The listing builds one solid part. Answer for the finished solid, in the listing's coordinates (mm). A direction names the side the tool comes from. Give positions to 0.01 mm unless a question says otherwise; leave off trailing zeros. Order: outer loops, then holes, each group sorted by start corner. A loop starts at its lowest first (then second) coordinate and runs counter-clockwise, first axis right, second up. Notation, with made-up numbers: (19.5, -35.75) - (69.5, -35.75) arc R22 ccw to (69.5, -17.75) - close; hole circle Ø10 at (53, 66.25). An arc over 180 degrees is marked (long way). Use a Markdown table: item, result. Add a question column.
1) The mould has two halves that part along X. Classify faces 4 (the face through (15, 0, 2)), 5 (the face through (13.953, 18.192, 2.348)), 6 (the face through (6.35, 2, 2)): released by +X, released by -X, zero draft, split by the parting line, or undercut.
2) Find section A-A, the plane y = 32. Determine the outline of the cut face in (x, z), plus the area to 3 significant figures.
3) Find section D-D, the plane y = 17.5. Determine the outline of the cut face in (x, z), plus the area to 3 significant figures.
4) Flat-ended cylindrical pins translate along their axes: pin 1 (2.5 mm diameter, centred on y = 30.5, z = 2, fed in from +X); pin 2 (1.4 mm diameter, centred on x = 0.5, z = 3, fed in from +Y); pin 3 (1.4 mm diameter, centred on y = 3, z = 2.5, fed in from -X). Find the tip coordinate at first contact, or state that the pin passes through.
5) Find section B-B, the plane z = 3.35. Determine the outline of the cut face in (x, y), plus the area to 3 significant figures.
6) For faces 1 (the face through (-6.35, 2, 2)), 2 (the face through (0, 25.722, 2)), 3 (the face through (-15, 0, 2)), determine the directions among +Z, -Z, +X, -X, +Y, -Y from which every point of the face is accessible in a straight line to the end or side of a thin tool.
7) Straight lines are drawn through the part: line 1 (Y direction, x = -1.5, z = 1.5); line 2 (X direction, y = 30, z = 0.25); line 3 (X direction, y = 27, z = 2.05). For each, find the intervals that lie inside material, in ascending order.
8) Find section C-C, the plane x = 1. Determine the outline of the cut face in (y, z), plus the area to 3 significant figures.
from build123d import *

# Parameters (mm, degrees)
BOSS_EXTRUDE1_DEPTH = 4.7625
CUT_EXTRUDE1_DEPTH  = 50.252795761
SKETCH4_W           = 4.7625
SKETCH4_H           = 4.7625
CUT_EXTRUDE2_DEPTH  = 10.16


with BuildPart() as part:
    # Sketch1 → Boss-Extrude1 (new body)
    with BuildSketch(Plane.XY):
        Polygon((0, 42.527367988), (24.384, 0), (-24.384, 0), align=None)
    extrude(amount=BOSS_EXTRUDE1_DEPTH)

    # Sketch2 → Cut-Extrude1 (cut, through all)
    with BuildSketch(Plane.XY.offset(4.7625)):
        Polygon((0, 0), (-6.35, 0), (-6.35, 4.7625), (6.35, 4.7625), (6.35, 0), align=None)
        Polygon((0, 42.527367988), (-3.81, 35.88246674), (3.81, 35.88246674), align=None)
    extrude(amount=-CUT_EXTRUDE1_DEPTH, mode=Mode.SUBTRACT)

    # Sketch4 → Cut-Extrude2 (cut)
    with BuildSketch(Plane(origin=(0, 35.88246674, 0), x_dir=(1, 0, 0), z_dir=(0, 1, 0))):
        with Locations((0, -2.38125)):
            Rectangle(SKETCH4_W, SKETCH4_H)
    extrude(amount=-CUT_EXTRUDE2_DEPTH, mode=Mode.SUBTRACT)


solid = part.part
The answers:
| question | item | result |
|---|---|---|
| 1 | face 4 | zero draft |
| 1 | face 5 | released by +X |
| 1 | face 6 | undercut |
| 2 | outline | (-6.04, 0) - (-2.38, 0) - (-2.38, 4.76) - (-6.04, 4.76) - close; (2.38, 0) - (6.04, 0) - (6.04, 4.76) - (2.38, 4.76) - close |
| 2 | area | 34.8 mm2 |
| 3 | outline | (-14.35, 0) - (14.35, 0) - (14.35, 4.76) - (-14.35, 4.76) - close |
| 3 | area | 137 mm2 |
| 4 | pin 1 | x = 7.61 |
| 4 | pin 2 | y = 25.72 |
| 4 | pin 3 | x = -23.07 |
| 5 | outline | (-24.38, 0) - (-6.35, 0) - (-6.35, 4.76) - (6.35, 4.76) - (6.35, 0) - (24.38, 0) - (3.81, 35.88) - (2.38, 35.88) - (2.38, 25.72) - (-2.38, 25.72) - (-2.38, 35.88) - (-3.81, 35.88) - close |
| 5 | area | 903 mm2 |
| 6 | face 1 | +Z, -Z, -Y |
| 6 | face 2 | +Z, -Z, +Y |
| 6 | face 3 | +Z, -Z, +X, -X, -Y |
| 7 | line 1 | 4.76 to 25.72 |
| 7 | line 2 | -7.18 to -2.38, 2.38 to 7.18 |
| 7 | line 3 | -8.9 to -2.38, 2.38 to 8.9 |
| 8 | outline | (4.76, 0) - (25.72, 0) - (25.72, 4.76) - (4.76, 4.76) - close |
| 8 | area | 99.8 mm2 |
